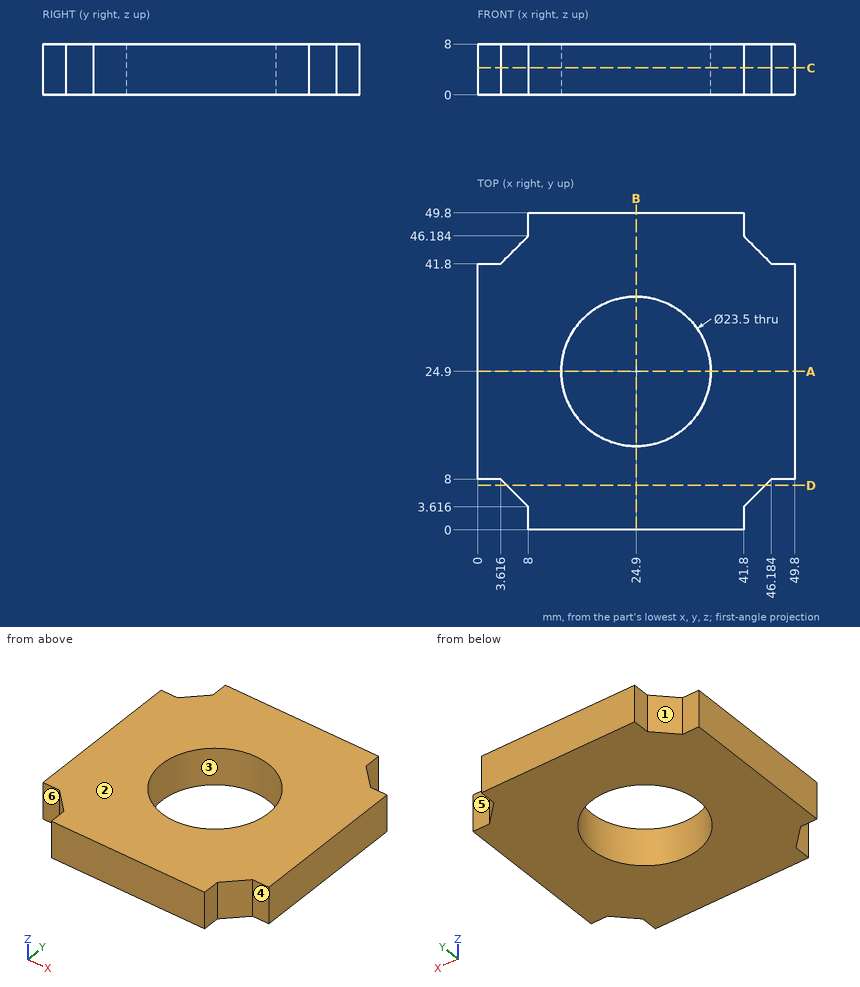
Geometry: see drawing. Coordinates: mm, zero at the bounding-box minimum. A direction names the side the tool comes from. Give positions to 0.01 mm unless a question says otherwise; leave off trailing zeros. Loops run counter-clockwise (first coordinate to the right, second up) from the corner with the lowest first, then second, coordinate; pieces in that order, holes last. Notation, with made-up numbers: M -3.5,13 L 8.5,13 A22 ccw 8.5,38 Z; hole C 59,47.5 d11. An arc over 180 degrees is marked long. Answer as CSV lines item,"result". Start each with the question number.
1. Pin query (flat end, axial travel): P1, Ø1.8, axis at x = 48.5, z = 4.5, coming from the -Y side; P2, Ø4, axis at x = 1, z = 2.5, coming from the +Y side; P3, Ø1.8, axis at y = 1.5, z = 3.5, coming from the -X side. Return the tip coordinate at first contact, or that it passes through.
2. Line query: L1, parallel to Y at x = 24.9, z = 6; L2, parallel to Y at x = 19.5, z = 7.75 (1 decimal); L3, parallel to X at y = 33.5, z = 1.25 (1 decimal). Output: solid intervals per line, ascending.
3. Section A-A on y = 24.9. Return loops of the section in (x, z).
4. Section D-D on y = 7. Return loops of the section in (x, z).
5. Section C-C on z = 4.25. Return loops of the section in (x, y), plus the area to 3 significant figures.
6. Pull-direction query (X, two-part tool) for the marked faces 1, 2 and 3; classes: released by +X, released by -X, zero draft, split by the parting line, or undercut.
7. Reachability of the marked faces 4, 5 and 6 from +Z, -Z, +X, -X, +Y, -Y: full face, straight path, thin tool, end or side. Return the list, or none.
Computed values:
1,P1,"stops at y = 8"
1,P2,"stops at y = 41.8"
1,P3,"stops at x = 8"
2,L1,"y = 0 to 13.15, 36.65 to 49.8"
2,L2,"y = 0 to 14.5, 35.3 to 49.8"
2,L3,"x = 0 to 16.9, 32.9 to 49.8"
3,outline,"M 0,0 L 13.15,0 L 13.15,8 L 0,8 Z; M 36.65,0 L 49.8,0 L 49.8,8 L 36.65,8 Z"
4,outline,"M 4.62,0 L 45.18,0 L 45.18,8 L 4.62,8 Z"
5,outline,"M 0,8 L 3.62,8 L 8,3.62 L 8,0 L 41.8,0 L 41.8,3.62 L 46.18,8 L 49.8,8 L 49.8,41.8 L 46.18,41.8 L 41.8,46.18 L 41.8,49.8 L 8,49.8 L 8,46.18 L 3.62,41.8 L 0,41.8 Z; hole C 24.9,24.9 d23.5"
5,area,"1,830 mm²"
6,face 1,"released by -X"
6,face 2,"zero draft"
6,face 3,"undercut"
7,face 4,"+Z, -Z, +X, -Y"
7,face 5,"+Z, -Z, +X, +Y"
7,face 6,"+Z, -Z, -X, -Y"
